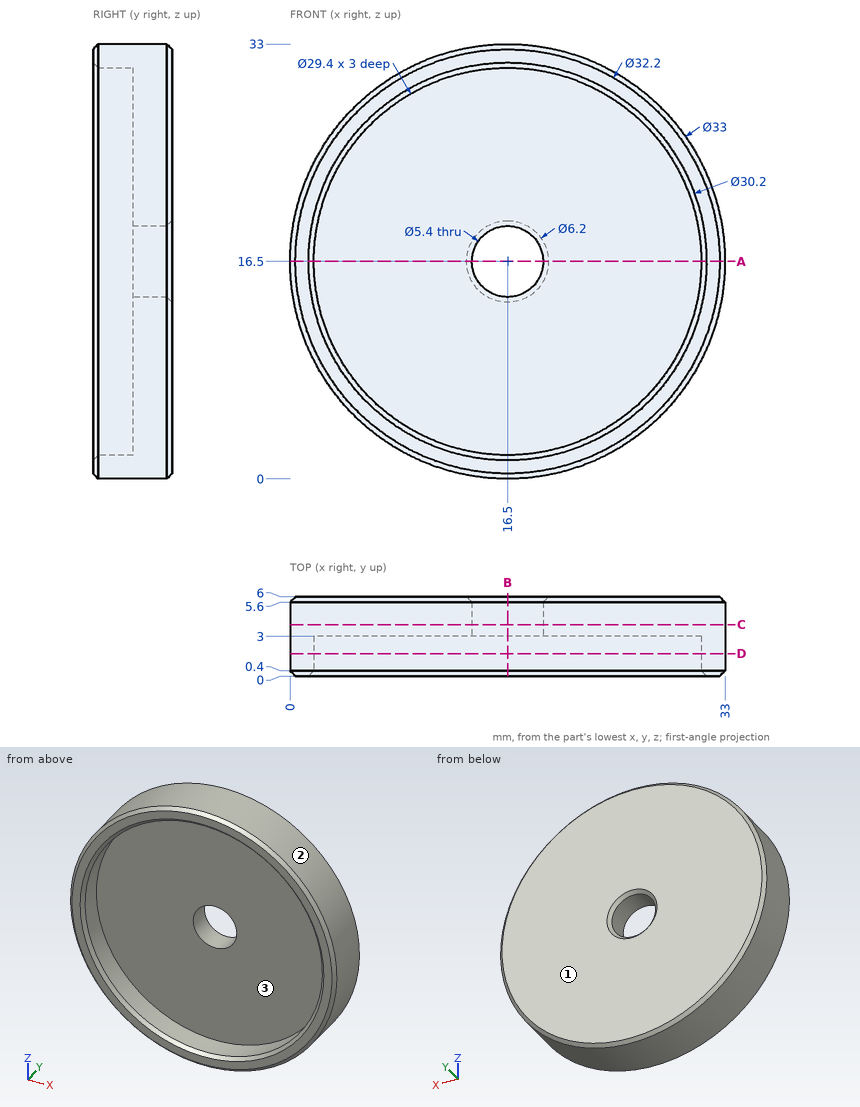
Here's the drawing with two shaded views (mm, measured from the low corner). I have some questions. Round coordinates to 2 decimals unless told otherwise and drop trailing zeros. Order: outer loops, then holes, each group sorted by start corner. A loop starts at its lowest first (then second) coordinate and runs counter-clockwise, first axis right, second up. Notation, with made-up numbers: M -34.5,44.25 L -5.5,44.25 A7 ccw -5.5,52.25 Z; hole C 4.5,-35.5 d8. An arc over 180 degrees is marked long. Use CSV: the item, a comma, the result in double quotes.
1) I need wall thicknesses on line 1 along X through (y, z) = (0.4, 17); line 2 along Y through (x, z) = (11.5, 28.5); line 3 along Z through (x, y) = (27.5, 1.35). Which ranges of each line are inside material? Lowest first, please. Write a range as [from, to].
Taken from the geometry:
line 1,"[0.01, 1.81], [31.19, 32.99]"
line 2,"[3, 6]"
line 3,"[4.2, 6.75], [26.25, 28.8]"
2) I want a section at D-D (y = 1.7). List the corners of the cut face in (x, z) for me, then the cut area to 3 significant figures.
Taken from the geometry:
outline,"C 16.5,16.5 d33; hole C 16.5,16.5 d29.4"
area,"176 mm^2"
3) I want a section at A-A (z = 16.5). List the corners of the cut face in (x, y) for me, then the cut area to 3 significant figures.
Taken from the geometry:
outline,"M 0,0.4 L 0.4,0 L 1.4,0 L 1.8,0.4 L 1.8,3 L 13.8,3 L 13.8,5.6 L 13.4,6 L 0.4,6 L 0,5.6 Z; M 19.2,3 L 31.2,3 L 31.2,0.4 L 31.6,0 L 32.6,0 L 33,0.4 L 33,5.6 L 32.6,6 L 19.6,6 L 19.2,5.6 Z"
area,"93.0 mm^2"
4) I want a section at C-C (y = 3.9). List the corners of the cut face in (x, z) for me, then the cut area to 3 significant figures.
Taken from the geometry:
outline,"C 16.5,16.5 d33; hole C 16.5,16.5 d5.4"
area,"832 mm^2"
5) If we mould it in two halves opening along X, with no side actions, what happens to the marked faces 1, 2 and 3? For each: pulls with the +X half, pulls with the -X half, needs draft (parallel to the pull), parting line crosses it, or undercut.
Taken from the geometry:
face 1,"needs draft"
face 2,"parting line crosses it"
face 3,"undercut"
6) I'm going to push flat-ended pins straight in: P1, Ø12, axis at x = 7.5, z = 25, coming from the -Y side; P2, Ø1.5, axis at x = 25.5, y = 1, coming from the -Z side; P3, Ø14.5, axis at x = 13.5, z = 14, coming from the -Y side; P4, Ø1.5, axis at y = 2, z = 18, coming from the +X side. Where does each tip first touch, or does it pass through?
Taken from the geometry:
P1,"y = 0"
P2,"z = 2.21"
P3,"y = 3"
P4,"x = 32.98"
7) I want a section at B-B (x = 16.5). List the corners of the cut face in (y, z) for me.
Taken from the geometry:
outline,"M 0,0.4 L 0.4,0 L 5.6,0 L 6,0.4 L 6,13.4 L 5.6,13.8 L 3,13.8 L 3,1.8 L 0.4,1.8 L 0,1.4 Z; M 0,31.6 L 0.4,31.2 L 3,31.2 L 3,19.2 L 5.6,19.2 L 6,19.6 L 6,32.6 L 5.6,33 L 0.4,33 L 0,32.6 Z"
